Read the model definition and answer for the solid it produces. Units are mm, in the model's axes. A direction names the side the tool comes from. Coordinates: 2 decimals unless noted, no trailing zeros. Write each loop counter-clockwise with the first axis right and the second up, starting at its lowest first coordinate (ties: lowest second). Pieces come first, ordered by that corner, then holes.
(1) The part is cut by section A-A, the plane y = -15. Determine the outline of the cut face in (x, z).
(2) Given pin 1 (16 mm diameter, centred on y = -21.5, z = 36, fed in from -X); pin 2 (12 mm diameter, centred on x = -27.5, y = -21, fed in from +Z); pin 3 (20 mm diameter, centred on x = -55.5, y = -19.5, fed in from -Z), each flat-ended and moving along its own axis, determine where each tip first touches the part or whether it passes through.
(3) Determine the mould class of faces 1 (the flat face through (-17.1, -4.6, 45)), 2 (the cylindrical face through (-42.05, -0.07, 5.46)), 3 (the flat face through (-100, 0, 23)) for opening direction X: pulls with the +X half, pulls with the -X half, needs draft (parallel to the pull), parting line crosses it, or undercut.
(4) The part is cut by section B-B, the plane y = -23. Determine the outline of the cut face in (x, z), and give its area (3 significant figures).
(5) Which of the six approach directions +Z, -Z, +X, -X, +Y, -Y give full straight-line access (tool end or side, diameter ignored) to faces 4 (the flat face through (-86.514, 0.07, 21.415)), 5 (the flat face through (-97.5, 3, 15)), 6 (the cylindrical face through (-79.38, -0.07, 28.8))?
(6) Straight lines are drawn through the part: line 1 along X through (y, z) = (-45, 28.5); line 2 along Z through (x, y) = (-80, -1.75); line 3 along Y through (x, z) = (-18, 40.5). For each, find the intervals that lie inside material, in ascending order.
Solid Edge part; units mm, degrees
sketch "Sketch1" plane through (0, 0, 0) normal (0, -1, 0) x (1, 0, 0)
  line L0 (10, 45) -> (10, 25)
  line L1 (-32.5, 25) -> (10, 25)
  line L2 (-32.5, 5) -> (-32.5, 25)
  arc A0 (-32.5, 5) -> (-47.5, 5) centre (-40, 5) cw
  line L3 (-47.5, 25) -> (-47.5, 5)
  line L4 (-82.9289, 25) -> (-47.5, 25)
  line L5 (-90, 17.9289) -> (-82.9289, 25)
  line L6 (-90, 10) -> (-90, 17.9289)
  line L7 (-100, 10) -> (-90, 10)
  line L8 (-100, 35) -> (-100, 10)
  line L9 (-90, 45) -> (-100, 35)
  line L10 (10, 45) -> (-90, 45)
  dimension "D1" = 90
extrude "Protrusion1" add sketch "Sketch1" along normal mid plane 10
sketch "Sketch2" plane through (0, 0, 0) normal (0, -1, 0) x (1, 0, 0)
  circle A0 centre (-80, 30) radius 1.35
extrude "ExtrudedCutout_3" cut sketch "Sketch2" along normal mid plane 29.2691
hole "Hole_1" at (-40, -5, 5) direction (0, 1, 0) diameter 4.2 end up to next
fillet "Round_7" radius 25 2 edges at (-47.5, 0, 25) (-32.5, 0, 25)
sketch "Sketch3" plane through (10, 0, 30) normal (1, 0, 0) x (0, 1, 0)
  line L0 (5, 15) -> (-55, 15)
  line L1 (-55, 15) -> (-55, -5)
  line L2 (-55, -5) -> (5, -5)
  line L3 (5, -5) -> (5, 15)
  dimension "D1" = 55
extrude "ExtrudedProtrusion_3" add sketch "Sketch3" against normal blind 20
fillet "Round_8" radius 10 2 edges at (-10, -55, 35) (10, -55, 35)
fillet "Round_9" radius 5 1 edges at (10, 5, 35)
sketch "Sketch4" plane through (-50, 5, 17.5) normal (0, 1, 0) x (1, 0, 0)
  line L0 (-47.5, 7.5) -> (-47.5, -0.5)
  line L1 (-47.5, -0.5) -> (-42.5, -0.5)
  line L2 (-42.5, -0.5) -> (-42.5, 7.5)
  line L3 (-42.5, 7.5) -> (-47.5, 7.5)
  dimension "D1" = 42.5
  dimension "D2" = 42.5
extrude "ExtrudedCutout_5" cut sketch "Sketch4" against normal blind 5
sketch "Sketch5" plane through (-65, -5, 17.5) normal (0, -1, 0) x (1, 0, 0)
  line L0 (-25, -7.5) -> (-35, -5.9162)
  line L1 (-35, -5.9162) -> (-35, -7.5)
  line L2 (-35, -7.5) -> (-25, -7.5)
extrude "ExtrudedCutout_6" cut sketch "Sketch5" against normal blind 31.7921
sketch "Sketch6" plane through (-8.75, -25, 25) normal (0, 0, -1) x (1, 0, 0)
  circle A0 centre (8.75, 20) radius 3
extrude "ExtrudedCutout_7" cut sketch "Sketch6" against normal blind 10
fillet "Round_11" radius 2 1 edges at (-3, -45, 25)
sketch "Sketch7" plane through (-40, -25, 35) normal (0, 0, 1) x (-1, 0, 0)
  line L0 (-30, 20) -> (39.282, -20)
  line L1 (39.282, -20) -> (-30, -20)
  line L2 (-30, -20) -> (-30, 20)
extrude "ExtrudedProtrusion_4" add sketch "Sketch7" along normal mid plane 10
properties material "PPA-CF"
Computed:
1. outline: (-61.96, 30) - (-10, 30) - (-10, 25) - (10, 25) - (10, 45) - (-10, 45) - (-10, 40) - (-61.96, 40) - close
2. pin 1: stops at x = -64.56
2. pin 2: stops at z = 40
2. pin 3: stops at z = 30
3. face 1: needs draft
3. face 2: undercut
3. face 3: pulls with the -X half
4. outline: (-48.11, 30) - (-10, 30) - (-10, 25) - (10, 25) - (10, 45) - (-10, 45) - (-10, 40) - (-48.11, 40) - close
4. area: 781 mm2
5. face 4: -Z, +Y, -Y
5. face 5: -Z, +Y
5. face 6: +Y
6. line 1: x = -10 to -3, 3 to 10
6. line 2: z = 25 to 28.65, 31.35 to 45
6. line 3: y = -5 to 5
